Here's how the part is built. I have some questions about the finished solid (model axes, mm). Coordinates: 2 decimals unless noted, no trailing zeros. Loops run counter-clockwise (first coordinate to the right, second up) from the corner with the lowest first, then second, coordinate; pieces in that order, holes last. Notation, with made-up numbers: (-8.75, 13) -> (-3.75, 13) arc R18 ccw to (-3.75, 33) -> close; hole circle Ø5 at (-5, 58.25). An arc over 180 degrees is marked (long way). Answer as a JSON object with one key per item and string values. Group by question number.
Q1. I need wall thicknesses on line 1 (Y direction, x = 0, z = 3.5); line 2 (X direction, y = 0, z = 4.25); line 3 (X direction, y = 110, z = 7). Which ranges of each line are inside material? Lowest first, please.
Q2. I'm going to push flat-ended pins straight in: pin 1 (3 mm diameter, centred on y = -34, z = 7, fed in from -X); pin 2 (0.7 mm diameter, centred on x = -137.5, y = 58, fed in from -Z); pin 3 (1 mm diameter, centred on x = -72, z = 8, fed in from -Y). Where does each tip first touch, or does it pass through?
Q3. I want a section at A-A on x = 79.5. Write out the boundary of the cut face in (y, z), then the cut area to 3 significant figures.
```python
from build123d import *

# Parameters (mm, degrees)
BOSS_EXTRU_1_DEPTH           = 9.5
BOSS_EXTRU_2_DEPTH           = 5
R_P_TITION_CIRCULAIRE1_COUNT = 31
R_P_TITION_CIRCULAIRE1_ANGLE = 343.6851996


with BuildPart() as part:
    # Esquisse1 → Boss.-Extru.1 (new body)
    with BuildSketch(Plane.XY):
        with BuildLine():
            Line((148.415801046, 5), (147.915516427, 5))
            ThreePointArc((147.915516427, 5), (-148, 0), (147.915516427, -5))
            Line((147.915516427, -5), (148.415801046, -5))
            ThreePointArc((148.415801046, -5), (-148.5, 0), (148.415801046, 5))
        make_face()
    extrude(amount=BOSS_EXTRU_1_DEPTH)

    # Esquisse2 → Boss.-Extru.2 (add)
    with BuildSketch(Plane.XY.offset(2.25)):
        Polygon((146.960409873, 24.517699499), (147.700328689, 19.572750546), (147.214129757, 19.5), (146.474210941, 24.444948953), align=None)
    boss_extru_2 = extrude(amount=BOSS_EXTRU_2_DEPTH)

    # Répétition circulaire1: Boss.-Extru.2 ×31 about axis
    r_p_tition_circulaire1_axis = Axis((0, 0, 0), (0, 0, 1))
    for i in range(1, R_P_TITION_CIRCULAIRE1_COUNT):
        add(boss_extru_2.rotate(r_p_tition_circulaire1_axis, i * R_P_TITION_CIRCULAIRE1_ANGLE / (R_P_TITION_CIRCULAIRE1_COUNT - 1)))


solid = part.part
```
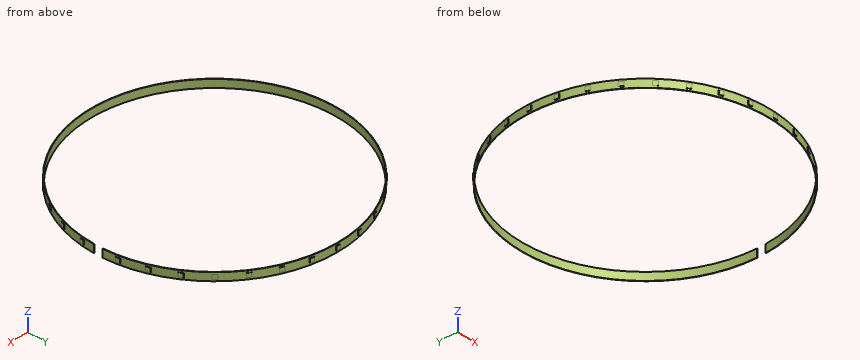
Result set:
{
 "1": {"line 1": "y = -148.5 to -148, 148 to 148.5", "line 2": "x = -148.97 to -148", "line 3": "x = -99.76 to -99.02, 99.02 to 99.76"},
 "2": {"pin 1": "stops at x = -145.4", "pin 2": "stops at z = 2.25", "pin 3": "stops at y = -130.15"},
 "3": {"outline": "(-125.43, 0) -> (-124.83, 0) -> (-124.83, 9.5) -> (-125.43, 9.5) -> close; (124.83, 0) -> (125.43, 0) -> (125.43, 9.5) -> (124.83, 9.5) -> close", "area": "11.3 mm²"}
}
